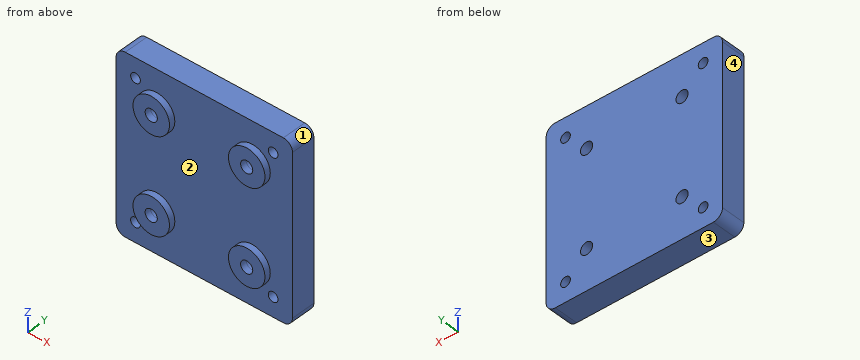
```python
from build123d import *

# Parameters (mm, degrees)
SZKIC2_R                    = 6
SZKIC2_R_2                  = 1.6
SZKIC2_R_3                  = 1.598649761
SZKIC2_R_4                  = 1.598671199
SZKIC2_R_5                  = 2
DODANIE_WYCI_GNI_CIE1_DEPTH = 8
SZKIC2_3_R                  = 6
SZKIC2_3_R_2                = 2
DODANIE_WYCI_GNI_CIE2_DEPTH = 2


with BuildPart() as part:
    # Szkic2 → Dodanie-wyci_gni_cie1 (new body)
    with BuildSketch(Plane(origin=(0, 0, 0), x_dir=(1, 0, 0), z_dir=(0, 1, 0))):
        with BuildLine():
            ThreePointArc((-76.341028527, -58.261863724), (-78.46234887, -57.383184068), (-79.341028527, -55.261863724))
            Line((-79.341028527, -55.261863724), (-79.341028527, -3.261863724))
            ThreePointArc((-79.341028527, -3.261863724), (-78.46234887, -1.140543381), (-76.341028527, -0.261863724))
            Line((-76.341028527, -0.261863724), (-24.341028527, -0.261863724))
            ThreePointArc((-24.341028527, -0.261863724), (-22.219708183, -1.140543381), (-21.341028527, -3.261863724))
            Line((-21.341028527, -3.261863724), (-21.341028527, -55.261863724))
            ThreePointArc((-21.341028527, -55.261863724), (-22.219708183, -57.383184068), (-24.341028527, -58.261863724))
            Line((-24.341028527, -58.261863724), (-76.341028527, -58.261863724))
        make_face()
        with Locations((-34.646028527, -44.956863724)):
            Circle(SZKIC2_R, mode=Mode.SUBTRACT)
        with Locations((-66.036028527, -44.956863724)):
            Circle(SZKIC2_R, mode=Mode.SUBTRACT)
        with Locations((-34.646028527, -13.566863724)):
            Circle(SZKIC2_R, mode=Mode.SUBTRACT)
        with Locations((-66.036028527, -13.566863724)):
            Circle(SZKIC2_R, mode=Mode.SUBTRACT)
        with Locations((-72.966028527, -51.886863724)):
            Circle(SZKIC2_R_2, mode=Mode.SUBTRACT)
        with Locations((-27.716028527, -51.886863724)):
            Circle(SZKIC2_R_3, mode=Mode.SUBTRACT)
        with Locations((-27.716028527, -6.636863724)):
            Circle(SZKIC2_R_2, mode=Mode.SUBTRACT)
        with Locations((-72.966028527, -6.636863724)):
            Circle(SZKIC2_R_4, mode=Mode.SUBTRACT)
        with Locations((-34.646028527, -13.566863724)):
            Circle(SZKIC2_R)
        with Locations((-34.646028527, -13.566863724)):
            Circle(SZKIC2_R_5, mode=Mode.SUBTRACT)
        with Locations((-66.036028527, -13.566863724)):
            Circle(SZKIC2_R)
        with Locations((-66.036028527, -13.566863724)):
            Circle(SZKIC2_R_5, mode=Mode.SUBTRACT)
        with Locations((-34.646028527, -44.956863724)):
            Circle(SZKIC2_R)
        with Locations((-34.646028527, -44.956863724)):
            Circle(SZKIC2_R_5, mode=Mode.SUBTRACT)
        with Locations((-66.036028527, -44.956863724)):
            Circle(SZKIC2_R)
        with Locations((-66.036028527, -44.956863724)):
            Circle(SZKIC2_R_5, mode=Mode.SUBTRACT)
    extrude(amount=DODANIE_WYCI_GNI_CIE1_DEPTH)

    # Szkic2_3 → Dodanie-wyci_gni_cie2 (add)
    with BuildSketch(Plane(origin=(0, 0, 0), x_dir=(1, 0, 0), z_dir=(0, 1, 0))):
        with Locations((-66.036028527, -13.566863724)):
            Circle(SZKIC2_3_R)
        with Locations((-66.036028527, -13.566863724)):
            Circle(SZKIC2_3_R_2, mode=Mode.SUBTRACT)
        with Locations((-34.646028527, -13.566863724)):
            Circle(SZKIC2_3_R)
        with Locations((-34.646028527, -13.566863724)):
            Circle(SZKIC2_3_R_2, mode=Mode.SUBTRACT)
        with Locations((-66.036028527, -44.956863724)):
            Circle(SZKIC2_3_R)
        with Locations((-66.036028527, -44.956863724)):
            Circle(SZKIC2_3_R_2, mode=Mode.SUBTRACT)
        with Locations((-34.646028527, -44.956863724)):
            Circle(SZKIC2_3_R)
        with Locations((-34.646028527, -44.956863724)):
            Circle(SZKIC2_3_R_2, mode=Mode.SUBTRACT)
    extrude(amount=-DODANIE_WYCI_GNI_CIE2_DEPTH)


solid = part.part
```
Build history of the part. All positions in model axes, mm. Face numbers are marked on the shaded views. Round coordinates to 2 decimals unless told otherwise and drop trailing zeros. Write each loop counter-clockwise with the first axis right and the second up, starting at its lowest first coordinate (ties: lowest second). Pieces come first, ordered by that corner, then holes. Notation, with made-up numbers: (-15, 18.5) - (-3, 18.5) arc R29 ccw to (-3, 45.5) - close; hole circle Ø1 at (-13.5, -22). An arc over 180 degrees is marked (long way). Write each question's results on one line, items separated by ' | '. Start each with the question number.
Item 1: Drop a flat-ended pin along its axis: P1, Ø3.5, axis at x = -72.97, z = 6.64, coming from the -Y side. Give the stop position or say it passes through.
Item 2: Saw through at B-B (y = 7.25). State how many separate pieces and enclosed holes the cut face has, and give its area (3 significant figures).
Item 3: Saw through at A-A (x = -27.5). Write the cut outline in (y, z).
Item 4: Saw through at C-C (z = 34). Write the cut outline in (x, y), and give its area (3 significant figures).
Item 5: Wall check: L1, parallel to Z at x = -67.5, y = 5.25; L2, parallel to X at y = 0.75, z = 14; L3, parallel to Z at x = -34, y = 3. Give the ranges that are in metal, low to high. Write a range as [from, to].
Item 6: Saw through at D-D (x = -46). Write the cut outline in (y, z), and give its area (3 significant figures).
Item 7: Mould opens along Z. For the marked faces 1, 2, 3 and 4 say: pulls with the +Z half, pulls with the -Z half, needs draft (parallel to the pull), parting line crosses it, or undercut.
Results are:
1) P1: stops at y = 0
2) separate pieces: 1 | enclosed holes: 8 | area: 3,270 mm²
3) outline: (0, 0.26) - (8, 0.26) - (8, 5.05) - (0, 5.05) - close; (0, 8.22) - (8, 8.22) - (8, 50.3) - (0, 50.3) - close; (0, 53.47) - (8, 53.47) - (8, 58.26) - (0, 58.26) - close
4) outline: (-79.34, 0) - (-21.34, 0) - (-21.34, 8) - (-79.34, 8) - close | area: 464 mm²
5) L1: z = [0.26, 12.2], [14.93, 43.59], [46.32, 58.26] | L2: x = [-79.34, -67.99], [-64.08, -36.6], [-32.69, -21.34] | L3: z = [0.26, 11.67], [15.46, 43.06], [46.85, 58.26]
6) outline: (0, 0.26) - (8, 0.26) - (8, 58.26) - (0, 58.26) - close | area: 464 mm²
7) face 1: pulls with the +Z half | face 2: undercut | face 3: pulls with the -Z half | face 4: needs draft
